Read the model definition and answer for the solid it produces. Units are mm, in the model's axes. Face numbers are marked on the shaded views. A direction names the side the tool comes from. Round coordinates to 2 decimals unless told otherwise and drop trailing zeros. Order: outer loops, then holes, each group sorted by start corner. A loop starts at its lowest first (then second) coordinate and runs counter-clockwise, first axis right, second up. Notation, with made-up numbers: (14, 25.5) -> (48, 25.5) arc R25 ccw to (48, 50.5) -> close; hole circle Ø4 at (11.5, 60.25). An arc over 180 degrees is marked (long way). Use a Markdown table: item, result. Add a question column.
1. Given pin 1 (9.5 mm diameter, centred on x = 10.5, z = 38.5, fed in from +Y); pin 2 (9.5 mm diameter, centred on y = 35, z = 26.5, fed in from +X); pin 3 (11 mm diameter, centred on y = 35.5, z = 25, fed in from -X); pin 4 (6.5 mm diameter, centred on y = 13, z = 16, fed in from -X), each flat-ended and moving along its own axis, determine where each tip first touches the part or whether it passes through.
2. Section B-B, the plane z = 16 is taken. Give the vertices of the cut face in (x, y).
3. For the marked faces 1, 2 and 3, determine the directions among +Z, -Z, +X, -X, +Y, -Y from which every point of the face is accessible in a straight line to the end or side of a thin tool.
4. Section A-A, the plane x = 9 is taken. Give the vertices of the cut face in (y, z), then the cut area to 3 significant figures.
5. Section D-D, the plane z = 26.5 is taken. Give the vertices of the cut face in (x, y), then the cut area to 3 significant figures.
6. Section C-C, the plane y = 14 is taken. Give the vertices of the cut face in (x, z), then the cut area to 3 significant figures.
7. Consider L1, parallel to Z at x = 9, y = 1.35; L2, parallel to Z at x = 9, y = 2.5; L3, parallel to Y at x = -0.3, z = 26.5. Determine where each line is inside the solid, lowest interval first. Write a range as [from, to].
```python
from build123d import *

# Parameters (mm, degrees)
SM_BASE_FLANGE_1_DEPTH    = 53
SKETCH_7_R                = 9
SKETCH_7_R_2              = 6
EXTRUDE_1_DEPTH           = 4
SKETCH_8_R                = 6
SKETCH_8_R_2              = 5
EXTRUDE_2_DEPTH           = 1
HOLE_WIZARD_1_D           = 4.6
HOLE_WIZARD_1_CBORE_D     = 8
HOLE_WIZARD_1_CBORE_DEPTH = 1
HOLE_WIZARD_2_D           = 5
HOLE_WIZARD_2_DEPTH       = 3
HOLE_WIZARD_2_CBORE_D     = 8
HOLE_WIZARD_2_CBORE_DEPTH = 1
HOLE_WIZARD_2_TIP         = 1.502151548
FILLET_1_R                = 3
CHAMFER_1_SIZE            = 1


# Read off the part's stored shape, not the designer's step: 基体-法兰1
with BuildPart() as part:
    # 基体-法兰1 outline → 基体-法兰1 (new body)
    with BuildSketch(Plane.XY):
        with BuildLine():
            Line((3, 3), (3, 62))
            Line((3, 62), (0, 62))
            Line((0, 62), (0, 3))
            ThreePointArc((0, 3), (0.878679656, 0.878679656), (3, 0))
            Line((3, 0), (15, 0))
            Line((15, 0), (15, 3))
            Line((15, 3), (3, 3))
        make_face()
    extrude(amount=SM_BASE_FLANGE_1_DEPTH)

    # 草图7 → 凸台-拉伸1 (add)
    with BuildSketch(Plane.ZY):
        with Locations((26.5, 35)):
            Circle(SKETCH_7_R)
        with Locations((26.5, 35)):
            Circle(SKETCH_7_R_2, mode=Mode.SUBTRACT)
    extrude(amount=EXTRUDE_1_DEPTH)

    # 草图8 → 凸台-拉伸2 (add)
    with BuildSketch(Plane.ZY):
        with Locations((26.5, 35)):
            Circle(SKETCH_8_R)
        with Locations((26.5, 35)):
            Circle(SKETCH_8_R_2, mode=Mode.SUBTRACT)
    extrude(amount=EXTRUDE_2_DEPTH)

    # 打孔尺寸(%根据)内六角圆柱头螺钉的类型1 (through all)
    with Locations(Plane(origin=(0, 3, 0), x_dir=(1, 0, 0), z_dir=(0, 1, 0))):
        with Locations((9, -6), (9, -47)):
            CounterBoreHole(HOLE_WIZARD_1_D / 2, HOLE_WIZARD_1_CBORE_D / 2, HOLE_WIZARD_1_CBORE_DEPTH)

    # 打孔尺寸(%根据)内六角圆柱头螺钉的类型2
    with Locations(Plane(origin=(3, 0, 0), x_dir=(0, 0, -1), z_dir=(1, 0, 0))):
        with Locations((-37, 13), (-16, 13)):
            CounterBoreHole(HOLE_WIZARD_2_D / 2, HOLE_WIZARD_2_CBORE_D / 2, HOLE_WIZARD_2_CBORE_DEPTH, depth=HOLE_WIZARD_2_DEPTH)
            with Locations((0, 0, -(HOLE_WIZARD_2_DEPTH + HOLE_WIZARD_2_TIP / 2))):  # 118° drill point
                Cone(0, HOLE_WIZARD_2_D / 2, HOLE_WIZARD_2_TIP, mode=Mode.SUBTRACT)

    # 圆角1
    fillet_1_edges = [part.edges().sort_by_distance(p)[0] for p in [
        (1.5, 62, 0),
        (1.5, 62, 53),
    ]]
    fillet(fillet_1_edges, radius=FILLET_1_R)

    # 倒角1
    chamfer_1_edges = [part.edges().sort_by_distance(p)[0] for p in [
        (-4, 35, 20.5),
    ]]
    chamfer(chamfer_1_edges, length=CHAMFER_1_SIZE)


solid = part.part
```
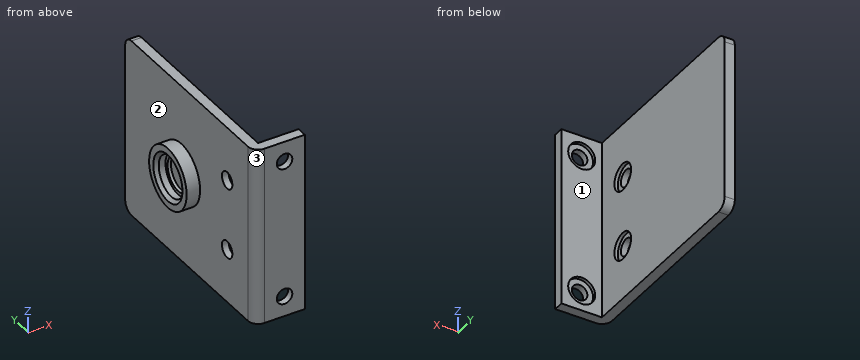
Verdict:
| question | item | result |
|---|---|---|
| 1 | pin 1 | stops at y = 3 |
| 1 | pin 2 | stops at x = 3 |
| 1 | pin 3 | stops at x = -4 |
| 1 | pin 4 | stops at x = 0 |
| 2 | outline | (0, 3) arc R3 ccw to (3, 0) -> (15, 0) -> (15, 3) -> (3, 3) -> (3, 9) -> (2, 9) -> (2, 10.5) -> (0, 10.5) -> close; (0, 15.5) -> (2, 15.5) -> (2, 17) -> (3, 17) -> (3, 62) -> (0, 62) -> close |
| 3 | face 1 | +Z, -Z, +X, +Y |
| 3 | face 2 | -X |
| 3 | face 3 | +Z, -Z, -X, -Y |
| 4 | outline | (0, 0) -> (3, 0) -> (3, 2) -> (2, 2) -> (2, 3.7) -> (0, 3.7) -> close; (0, 8.3) -> (2, 8.3) -> (2, 10) -> (3, 10) -> (3, 43) -> (2, 43) -> (2, 44.7) -> (0, 44.7) -> close; (0, 49.3) -> (2, 49.3) -> (2, 51) -> (3, 51) -> (3, 53) -> (0, 53) -> close |
| 4 | area | 125 mm2 |
| 5 | outline | (-4, 26) -> (0, 26) -> (0, 3) arc R3 ccw to (3, 0) -> (15, 0) -> (15, 3) -> (3, 3) -> (3, 62) -> (0, 62) -> (0, 44) -> (-4, 44) -> (-4, 42) -> (-3, 41) -> (-1, 41) -> (-1, 40) -> (0, 40) -> (0, 30) -> (-1, 30) -> (-1, 29) -> (-3, 29) -> (-4, 28) -> close |
| 5 | area | 245 mm2 |
| 6 | outline | (0, 0) -> (3, 0) -> (3, 12.13) -> (2, 12.13) -> (2, 13.71) -> (0, 13.71) -> close; (0, 18.29) -> (2, 18.29) -> (2, 19.87) -> (3, 19.87) -> (3, 33.13) -> (2, 33.13) -> (2, 34.71) -> (0, 34.71) -> close; (0, 39.29) -> (2, 39.29) -> (2, 40.87) -> (3, 40.87) -> (3, 53) -> (0, 53) -> close |
| 6 | area | 125 mm2 |
| 7 | L1 | z = [0, 3.7], [8.3, 44.7], [49.3, 53] |
| 7 | L2 | z = [0, 2], [10, 43], [51, 53] |
| 7 | L3 | y = [26, 30], [40, 44] |
